from build123d import *

# Parameters (mm, degrees)
F0_R     = 6.35
F0_R_2   = 12.7
F1_DEPTH = 12.7


with BuildPart() as f1:
    # F0 (on Right) → F1 (new body)
    with BuildSketch(Plane.YZ):
        with BuildLine():
            Line((-192.497232, 31.555194), (-262.760009, 31.555194))
            ThreePointArc((-262.760009, 31.555194), (-219.475912, -12.035632), (-163.940978, -38.294806))
            Line((-163.940978, -38.294806), (-69.755258, -38.294806))
            ThreePointArc((-69.755258, -38.294806), (28.342708, 235.782988), (-262.760009, 234.755194))
            Line((-262.760009, 234.755194), (-192.497232, 234.755194))
            ThreePointArc((-192.497232, 234.755194), (9.822117, 133.155194), (-192.497232, 31.555194))
        make_face()
        with Locations((-148.598118, -25.594806)):
            Circle(F0_R, mode=Mode.SUBTRACT)
        with Locations((-179.797232, -5.636625)):
            Circle(F0_R_2, mode=Mode.SUBTRACT)
        with Locations((-85.098118, -25.594806)):
            Circle(F0_R, mode=Mode.SUBTRACT)
        with Locations((-61.33506, -8.774579)):
            Circle(F0_R_2, mode=Mode.SUBTRACT)
        with Locations((23.561913, 73.903331)):
            Circle(F0_R_2, mode=Mode.SUBTRACT)
        with Locations((-179.797232, 271.947013)):
            Circle(F0_R_2, mode=Mode.SUBTRACT)
        with Locations((23.561913, 192.407056)):
            Circle(F0_R_2, mode=Mode.SUBTRACT)
        with Locations((-61.33506, 275.084967)):
            Circle(F0_R_2, mode=Mode.SUBTRACT)
    extrude(amount=F1_DEPTH)


solid = f1.part
Design review of the part built by this model. Coordinates are the model's own, in mm. A direction names the side the tool comes from. Coordinates: 2 decimals unless noted, no trailing zeros. Write each loop counter-clockwise with the first axis right and the second up, starting at its lowest first coordinate (ties: lowest second). Pieces come first, ordered by that corner, then holes. Notation, with made-up numbers: (86, 51.25) - (100, 51.25) arc R17 ccw to (100, 58.25) - close; hole circle Ø8 at (-4.5, -2.75). An arc over 180 degrees is marked (long way). Use one line per item in the form item = value.
Q1. Consider section A-A (y = -225.5). Write out the cut boundary in (x, z), plus the area to 3 significant figures.
Taken from the geometry:
outline = (0, -7.58) - (12.7, -7.58) - (12.7, 31.56) - (0, 31.56) - close; (0, 234.76) - (12.7, 234.76) - (12.7, 273.89) - (0, 273.89) - close
area = 994 mm^2
Q2. Consider section B-B (x = 5). Count the separate pieces of the cut face and the enclosed holes in it, plus the area to 3 significant figures.
Taken from the geometry:
separate_pieces = 1
enclosed_holes = 8
area = 33,800 mm^2
Q3. Consider section C-C (z = 200). Write out the cut boundary in (x, y).
Taken from the geometry:
outline = (0, -9.25) - (12.7, -9.25) - (12.7, 13.38) - (0, 13.38) - close; (0, 33.74) - (12.7, 33.74) - (12.7, 47.91) - (0, 47.91) - close
Q4. Consider section D-D (y = -178.5). Write out the cut boundary in (x, z).
Taken from the geometry:
outline = (0, -33.61) - (12.7, -33.61) - (12.7, -18.27) - (0, -18.27) - close; (0, 7) - (12.7, 7) - (12.7, 22.5) - (0, 22.5) - close; (0, 243.81) - (12.7, 243.81) - (12.7, 259.31) - (0, 259.31) - close; (0, 284.58) - (12.7, 284.58) - (12.7, 299.92) - (0, 299.92) - close
Q5. Insertion check: pin 1 Ø11.5 at (y, z) = (-85.1, -25.59) entering from -X; pin 2 Ø14.5 at (y, z) = (-148.6, -25.59) entering from +X; pin 3 Ø1.5 at (x, z) = (2, 275.5) entering from +Y; pin 4 Ø3 at (x, y) = (4, -52.5) entering from -Z. Each pin has a flat end and moves straight along its axis. Give the tip position at first contact, or say it passes through.
Taken from the geometry:
pin_1 = through
pin_2 = 12.7
pin_3 = -9.31
pin_4 = -33.17
Q6. For probe 1 along Z at (x, y) = (1.25, -121.5); probe 2 along Z at (x, y) = (7.5, -120); probe 3 along Z at (x, y) = (9, -189.5), list the stretches that pass through material, from the lowest coordinate up.
Taken from the geometry:
probe_1 = -38.29 to 6.57, 259.74 to 310.89
probe_2 = -38.29 to 6.52, 259.79 to 310.93
probe_3 = -29.12 to -13.83, 2.56 to 29.39, 236.92 to 263.75, 280.14 to 295.43
Q7. Machinability: for faces 4 (the flat face through (6, -228, 234.755)), 5 (the cylindrical face through (6.26, 20.81, 180.01)), which of the approach directions +Z, -Z, +X, -X, +Y, -Y give a long, thin tool a straight path to every point of the face, cutting with its end or side? Answer none if there is none.
Taken from the geometry:
face_4 = +X, -X, -Y
face_5 = +X, -X
Q8. The part is to be moulded in two halves that separate along Y. For faces 1 (the flat face through (0, 6, 176)), 2 (the cylindrical face through (6.261, -220.181, -11.535)), 3 (the cylindrical face through (6.261, -168.066, 267.083)), say which applies: +Y half, -Y half, draft (parallel to the pull), parting line (faces both ways), or undercut.
Taken from the geometry:
face_1 = draft
face_2 = -Y half
face_3 = undercut
